Design review of the part built by this model. Coordinates are the model's own, in mm. Coordinates: 2 decimals unless noted, no trailing zeros. Loops run counter-clockwise (first coordinate to the right, second up) from the corner with the lowest first, then second, coordinate; pieces in that order, holes last. Notation, with made-up numbers: M 89.5,-24 L 119.5,-24 A8 ccw 119.5,-11 Z; hole C 40.5,59 d2. An arc over 180 degrees is marked long. One line per item, written item: value.
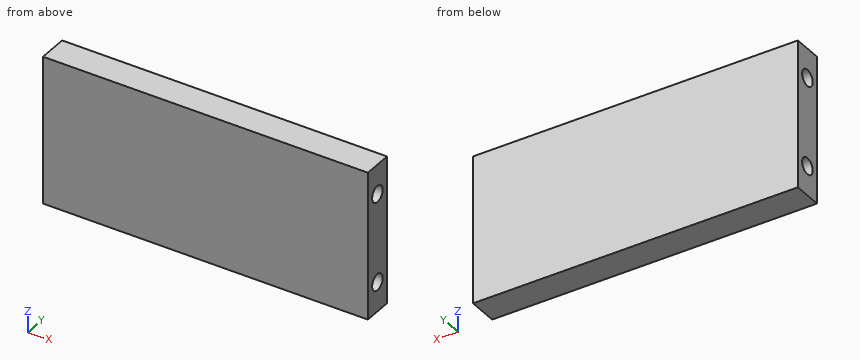
```python
from build123d import *

# Parameters (mm, degrees)
F0_W     = 69.85
F0_H     = 6.35
F1_DEPTH = 31.75
F2_R     = 1.75
F3_DEPTH = 12.7
F4_R     = 1.75
F5_DEPTH = 12.7


with BuildPart() as f1:
    # F0 (on Top) → F1 (new body)
    with BuildSketch(Plane.XY):
        with Locations((34.925, -3.175)):
            Rectangle(F0_W, F0_H)
    extrude(amount=F1_DEPTH)

    # F2 (on face) → F3 (cut)
    with BuildSketch(Plane.YZ.offset(69.85)):
        with Locations((-3.175, 25.4)):
            Circle(F2_R)
        with Locations((-3.175, 6.35)):
            Circle(F2_R)
    extrude(amount=-F3_DEPTH, mode=Mode.SUBTRACT)

    # F4 (on face) → F5 (cut)
    with BuildSketch(Plane(origin=(0, 0, 0), x_dir=(0, -1, 0), z_dir=(-1, 0, 0))):
        with Locations((3.175, 6.35)):
            Circle(F4_R)
        with Locations((3.175, 25.4)):
            Circle(F4_R)
    extrude(amount=-F5_DEPTH, mode=Mode.SUBTRACT)


solid = f1.part
```
(1) We need section C-C on z = 6.35. State the section outline as (x, y) points (3 decimals), then the cut area to 3 significant figures.
Reply:
outline: M 0,-6.35 L 69.85,-6.35 L 69.85,-4.925 L 57.15,-4.925 L 57.15,-1.425 L 69.85,-1.425 L 69.85,0 L 0,0 L 0,-1.425 L 12.7,-1.425 L 12.7,-4.925 L 0,-4.925 Z
area: 355 mm2
(2) Insertion check: pin 1 (1 mm diameter, centred on y = -3, z = 25.5, fed in from -X); pin 2 (1 mm diameter, centred on y = -2.5, z = 6, fed in from +X). Each pin has a flat end and moves straight along its axis. Give the tip position at first contact, or say it passes through.
Reply:
pin 1: stops at x = 12.7
pin 2: stops at x = 57.15
(3) We need section B-B on y = -4. State the section outline as (x, z) points.
Reply:
outline: M 0,0 L 69.85,0 L 69.85,4.81 L 57.15,4.81 L 57.15,7.89 L 69.85,7.89 L 69.85,23.86 L 57.15,23.86 L 57.15,26.94 L 69.85,26.94 L 69.85,31.75 L 0,31.75 L 0,26.94 L 12.7,26.94 L 12.7,23.86 L 0,23.86 L 0,7.89 L 12.7,7.89 L 12.7,4.81 L 0,4.81 Z
(4) We need section A-A on z = 24.5. State the section outline as (x, y) points.
Reply:
outline: M 0,-6.35 L 69.85,-6.35 L 69.85,-4.68 L 57.15,-4.68 L 57.15,-1.67 L 69.85,-1.67 L 69.85,0 L 0,0 L 0,-1.67 L 12.7,-1.67 L 12.7,-4.68 L 0,-4.68 Z
(5) To check wall thickness, follow line 1 along Y through (x, z) = (5, 6); line 2 along X through (y, z) = (-2.5, 25.5). State the ranges of each line that lie inside material, in increasing order. Write a range as [from, to].
Reply:
line 1: y = [-6.35, -4.89], [-1.46, 0]
line 2: x = [12.7, 57.15]
